from build123d import *

# Parameters (mm, degrees)
BOSS_EXTRUDE1_START = 0.1
SKETCH1_W           = 6.6
SKETCH1_H           = 6.6
BOSS_EXTRUDE1_DEPTH = 2.7
CUT_EXTRUDE1_START  = 0.1
SKETCH2_W           = 4
SKETCH2_H           = 3.6
CUT_EXTRUDE1_DEPTH  = 0.1
SKETCH3_W           = 1.6
SKETCH3_H           = 2.9
BOSS_EXTRUDE2_DEPTH = 0.8
FILLET1_R           = 0.5
FILLET2_R           = 0.1


with BuildPart() as part:
    # Sketch1 → Boss-Extrude1 (new body)
    with BuildSketch(Plane.XY.offset(BOSS_EXTRUDE1_START)):
        Rectangle(SKETCH1_W, SKETCH1_H)
    extrude(amount=BOSS_EXTRUDE1_DEPTH)

    # Sketch2 → Cut-Extrude1 (cut)
    with BuildSketch(Plane.XY.offset(CUT_EXTRUDE1_START)):
        with Locations((-3.3, 0)):
            Rectangle(SKETCH2_W, SKETCH2_H)
    cut_extrude1 = extrude(amount=CUT_EXTRUDE1_DEPTH, mode=Mode.SUBTRACT)

    # Mirror1: Cut-Extrude1 across plane
    add(cut_extrude1.mirror(Plane(origin=(0, 0, 0), x_dir=(0, 0, 1), z_dir=(1, 0, 0))), mode=Mode.SUBTRACT)

    # Sketch3 → Boss-Extrude2 (add)
    with BuildSketch(Plane.XY):
        with Locations((-2.7, 0)):
            Rectangle(SKETCH3_W, SKETCH3_H)
    boss_extrude2 = extrude(amount=BOSS_EXTRUDE2_DEPTH)

    # Mirror2: Boss-Extrude2 across plane
    add(boss_extrude2.mirror(Plane(origin=(0, 0, 0), x_dir=(0, 0, 1), z_dir=(1, 0, 0))))

    # Fillet1
    fillet1_edges = [part.edges().sort_by_distance(p)[0] for p in [
        (3.3, -3.3, 1.45),
        (-3.3, -3.3, 1.45),
        (-3.3, 3.3, 1.45),
        (3.3, 3.3, 1.45),
    ]]
    fillet(fillet1_edges, radius=FILLET1_R)

    # Fillet2
    fillet2_edges = [part.edges().sort_by_distance(p)[0] for p in [
        (3.5, -1.45, 0.4),
        (3.5, 0, 0.8),
        (3.5, 1.45, 0.4),
        (2.7, 1.45, 0),
        (1.9, 0, 0),
        (2.7, -1.45, 0),
        (3.5, 0, 0),
        (-2.7, -1.45, 0),
        (-1.9, 0, 0),
        (-2.7, 1.45, 0),
        (-3.5, 1.45, 0.4),
        (-3.5, 0, 0.8),
        (-3.5, -1.45, 0.4),
        (-3.5, 0, 0),
        (-2.6, 1.45, 0.2),
    ]]
    fillet(fillet2_edges, radius=FILLET2_R - 0.0001)  # a hair under: the kernel refuses the full size


solid = part.part
Read the model definition and answer for the solid it produces. Units are mm, in the model's axes. Give positions to 0.01 mm unless a question says otherwise; leave off trailing zeros. Write each loop counter-clockwise with the first axis right and the second up, starting at its lowest first coordinate (ties: lowest second). Pieces come first, ordered by that corner, then holes. Notation, with made-up numbers: (62, 56) -> (96, 56) arc R25 cw to (96, 90) -> close; hole circle Ø6 at (0.5, 4.25). An arc over 180 degrees is marked (long way). Answer as a JSON object with one key per item and string values. Group by question number.
1) Consider L1, parallel to X at y = 0.5, z = 2.1; L2, parallel to Z at x = 1, y = -1.5; L3, parallel to Y at x = -3, z = 2.4. Determine where each line is inside the solid, lowest interval first. Write a range as from..to.
2) This flat-tipped pin is pushed along its axis until it touches: P1, Ø1.5, axis at y = 2, z = 1.5, coming from the -X side. Where does it stop, or does it pass through?
3) Find section C-C (y = -1). Write down the section's boundary in (x, z), and give its area (3 significant figures).
4) Find section A-A (x = 1.5). Write down the section's boundary in (y, z).
5) The mould has two halves that part along X. Classify faces 1 (the flat face through (3, 0, 0)), 2 (the flat face through (0, 0, 0.1)): +X half, -X half, draft (parallel to the pull), parting line (faces both ways), or undercut.
6) Find section D-D (x = 2.5). Write down the section's boundary in (y, z).
7) Find section B-B (z = 1.45). Write down the section's boundary in (x, y).
Values follow:
{
 "1": {"L1": "x = -3.3..3.3", "L2": "z = 0.1..2.8", "L3": "y = -3.26..3.26"},
 "2": {"P1": "stops at x = -3.3"},
 "3": {"outline": "(-3.5, 0.1) arc R0.1 ccw to (-3.4, 0) -> (-2, 0) arc R0.1 ccw to (-1.9, 0.1) -> (-1.9, 0.2) -> (-1.3, 0.2) -> (-1.3, 0.1) -> (1.3, 0.1) -> (1.3, 0.2) -> (1.9, 0.2) -> (1.9, 0.1) arc R0.1 ccw to (2, 0) -> (3.4, 0) arc R0.1 ccw to (3.5, 0.1) -> (3.5, 0.7) arc R0.1 ccw to (3.4, 0.8) -> (3.3, 0.8) -> (3.3, 2.8) -> (-3.3, 2.8) -> (-3.3, 0.8) -> (-3.4, 0.8) arc R0.1 ccw to (-3.5, 0.7) -> close", "area": "18.3 mm2"},
 "4": {"outline": "(-3.3, 0.1) -> (-1.8, 0.1) -> (-1.8, 0.2) -> (1.8, 0.2) -> (1.8, 0.1) -> (3.3, 0.1) -> (3.3, 2.8) -> (-3.3, 2.8) -> close"},
 "5": {"face 1": "draft", "face 2": "undercut"},
 "6": {"outline": "(-3.3, 0.1) -> (-1.8, 0.1) -> (-1.8, 0.2) -> (-1.45, 0.2) -> (-1.45, 0.1) arc R0.1 ccw to (-1.35, 0) -> (1.35, 0) arc R0.1 ccw to (1.45, 0.1) -> (1.45, 0.2) -> (1.8, 0.2) -> (1.8, 0.1) -> (3.3, 0.1) -> (3.3, 2.8) -> (-3.3, 2.8) -> close"},
 "7": {"outline": "(-3.3, -2.8) arc R0.5 ccw to (-2.8, -3.3) -> (2.8, -3.3) arc R0.5 ccw to (3.3, -2.8) -> (3.3, 2.8) arc R0.5 ccw to (2.8, 3.3) -> (-2.8, 3.3) arc R0.5 ccw to (-3.3, 2.8) -> close"}
}
